```python
from build123d import *

# Parameters (mm, degrees)
F0_W      = 30
F0_H      = 10
F1_DEPTH  = 2
F2_W      = 30
F2_H      = 2
F3_DEPTH  = 6.5
F4_W      = 30
F4_H      = 10
F5_DEPTH  = 2
F6_R      = 2
F8_DEPTH  = 0.2
F10_DEPTH = 0.4
F12_DEPTH = 2
F14_DEPTH = 2
F15_R     = 1


with BuildPart() as f1:
    # F0 (on Top) → F1 (new body)
    with BuildSketch(Plane.XY):
        with Locations((15, 5)):
            Rectangle(F0_W, F0_H)
    extrude(amount=F1_DEPTH)

    # F2 (on face) → F3 (join)
    with BuildSketch(Plane.XY.offset(2)):
        with Locations((15, 1)):
            Rectangle(F2_W, F2_H)
    extrude(amount=F3_DEPTH)

    # F4 (on face) → F5 (join)
    with BuildSketch(Plane.XY.offset(8.5)):
        with Locations((15, 5)):
            Rectangle(F4_W, F4_H)
    extrude(amount=F5_DEPTH)

    # F6
    f6_edges = [f1.edges().sort_by_distance(p)[0] for p in [
        (30, 10, 9.5),
        (30, 10, 1),
        (0, 10, 9.5),
        (0, 10, 1),
    ]]
    fillet(f6_edges, radius=F6_R)

    # F7 (on face) → F8 (join)
    with BuildSketch(Plane.XY.offset(2)):
        with BuildLine():
            Line((28, 10), (2, 10))
            ThreePointArc((2, 10), (0.5857864376, 9.4142135624), (0, 8))
            Line((0, 8), (30, 8))
            ThreePointArc((30, 8), (29.4142135624, 9.4142135624), (28, 10))
        make_face()
    extrude(amount=F8_DEPTH)

    # F9 (on face) → F10 (join)
    with BuildSketch(Plane(origin=(0, 0, 8.5), x_dir=(1, 0, 0), z_dir=(0, 0, -1))):
        with BuildLine():
            ThreePointArc((0, -8), (0.5857864376, -9.4142135624), (2, -10))
            Line((2, -10), (28, -10))
            ThreePointArc((28, -10), (29.4142135624, -9.4142135624), (30, -8))
            Line((30, -8), (0, -8))
        make_face()
    extrude(amount=F10_DEPTH)

    # F11 (on face) → F12 (join, through all)
    with BuildSketch(Plane.XY.offset(10.5)):
        with BuildLine():
            Line((25, 0), (15, 0))
            Line((15, 0), (5, 0))
            ThreePointArc((5, 0), (15, -10), (25, 0))
        make_face()
    extrude(amount=-F12_DEPTH)

    # F13 (on face) → F14 (join, through all)
    with BuildSketch(Plane(origin=(0, 0, 0), x_dir=(1, 0, 0), z_dir=(0, 0, -1))):
        with BuildLine():
            ThreePointArc((25, 0), (15, 10), (5, 0))
            Line((5, 0), (25, 0))
        make_face()
    extrude(amount=-F14_DEPTH)

    # F15
    f15_edges = [f1.edges().sort_by_distance(p)[0] for p in [
        (15, 0, 2),
        (15, 0, 8.5),
        (5, 0, 9.5),
        (5, 0, 1),
        (25, 0, 9.5),
        (30, 0, 5.25),
        (0, 0, 5.25),
        (15, 2, 2),
        (15, 2, 8.5),
        (25, 0, 1),
    ]]
    fillet(f15_edges, radius=F15_R)


solid = f1.part
```
Can you work these out from the model? Positions are in its coordinate system, mm. A direction names the side the tool comes from. Coordinates: 2 decimals unless noted, no trailing zeros. Write each loop counter-clockwise with the first axis right and the second up, starting at its lowest first coordinate (ties: lowest second). Pieces come first, ordered by that corner, then holes. Notation, with made-up numbers: M 12.5,70 L 36.5,70 A20 ccw 36.5,101 Z; hole C -10.5,-29.5 d1. An arc over 180 degrees is marked long. Write item = value, one per line. Start each with the question number.
Q1. I'm going to push flat-ended pins straight in: pin 1 (1.5 mm diameter, centred on x = 20, z = 6, fed in from -Y); pin 2 (1.5 mm diameter, centred on y = -1, z = 8.5, fed in from +X); pin 3 (3 mm diameter, centred on y = -3, z = 1, fed in from +X). Where does each tip first touch, or does it pass through?
Q2. If we section it at C-C, the plane x = 12: Write out the boundary of the cut face in (y, z).
Q3. Thinking about a two-plate mould opening in Y: for faces 1 (the face through (15, 2, 10.5)), 2 (the face through (4.71, -0.25, 1.19)), 3 (the face through (15, 10, 1)), 4 (the face through (15, 6, 2)), which applies, released by +Y, released by -Y, zero draft, split by the parting line, or undercut?
Q4. If we section it at B-B, the plane z = 1.25: Write out the boundary of the cut face in (x, y).
Q5. If we section it at A-A, the plane y = 3.5: Write out the boundary of the cut face in (x, z), then the cut area to 3 significant figures.
Q6. On a 3-axis mill with a long thin cutter (end or side, diameter ignored), from which of +Z, -Z, +X, -X, +Y, -Y can I reach the whole of each face in a straight line? I mean faces 5 (the face through (15, 9, 8.1)), 6 (the face through (15, 6, 8.5)), 7 (the face through (15, 0, 5)), 8 (the face through (0, 1.3, 5.2)), 9 (the face through (15.153, -0.285, 2.301)). Say none if no direction works.
Q7. If we section it at D-D, the plane y = -7.5: Write out the boundary of the cut face in (x, z).
Q8. If I drill on L1, parallel to Z at x = 6.5, y = 6.25; L2, parallel to Y at x = 17.25, z = 3.25; L3, parallel to Z at x = 5.25, y = -0.5, over which ranges is the centre line in solid material (lowest first)? Write a range as [from, to].
Check sheet entries:
q1.pin_1 = 0
q1.pin_2 = 25.29
q1.pin_3 = 24.89
q2.outline = M -9.54,0 L 10,0 L 10,2.2 L 8,2.2 L 8,2 L 3,2 A1 cw 2,3 L 2,7.5 A1 cw 3,8.5 L 8,8.5 L 8,8.1 L 10,8.1 L 10,10.5 L -9.54,10.5 L -9.54,8.5 L -1,8.5 A1 cw 0,7.5 L 0,3 A1 cw -1,2 L -9.54,2 Z
q3.face_1 = zero draft
q3.face_2 = released by -Y
q3.face_3 = released by +Y
q3.face_4 = undercut
q4.outline = M 0,1 A1 ccw 1,0 L 4.05,0 A1 cw 5.04,-0.91 A10 ccw 24.96,-0.91 A1 cw 25.95,0 L 29,0 A1 ccw 30,1 L 30,8 A2 ccw 28,10 L 2,10 A2 ccw 0,8 Z
q5.outline = M 0,0 L 30,0 L 30,2 L 0,2 Z; M 0,8.5 L 30,8.5 L 30,10.5 L 0,10.5 Z
q5.area = 120 mm²
q6.face_5 = +X, -X, +Y
q6.face_6 = +X, -X
q6.face_7 = -Y
q6.face_8 = +Z, -Z, -X, +Y, -Y
q6.face_9 = +X, -X, -Y
q7.outline = M 8.39,0 L 21.61,0 L 21.61,2 L 8.39,2 Z; M 8.39,8.5 L 21.61,8.5 L 21.61,10.5 L 8.39,10.5 Z
q8.L1 = [0, 2], [8.5, 10.5]
q8.L2 = [0, 2]
q8.L3 = [0, 2.13], [8.37, 10.5]
